For this review, take the finished solid that the model builds, in its own axes (mm). A direction names the side the tool comes from. Coordinates: 2 decimals unless noted, no trailing zeros. Loops run counter-clockwise (first coordinate to the right, second up) from the corner with the lowest first, then second, coordinate; pieces in that order, holes last. Notation, with made-up numbers: (1, 28) - (34, 28) arc R30 ccw to (34, 67) - close; hole circle Ø9 at (28, 69). An arc over 180 degrees is marked (long way). Answer as a JSON object with one key per item and string values. Group by question number.
Item 1: We need section B-B (y = -6). Give the boundary of the cut face in (x, z).
Item 2: We need section D-D (y = 9). Give the boundary of the cut face in (x, z).
Item 3: To check wall thickness, follow line 1 (X direction, y = 0, z = 5.2); line 2 (X direction, y = -10, z = 4.15); line 3 (Y direction, x = 0, z = 8.25). State the ranges of each line that lie inside material, in increasing order.
Item 4: Clearance check with flat-ended pins moving along their axes: pin 1 (5.5 mm diameter, centred on x = -27, y = 7.5, fed in from -Z); pin 2 (1 mm diameter, centred on y = -17.5, z = 6, fed in from -X); pin 3 (0.5 mm diameter, centred on x = 12.5, z = 4, fed in from -Y); pin 4 (10 mm diameter, centred on x = -11.5, y = -6.5, fed in from +Z). State where each tip first meets the part, or that it passes through.
Item 5: We need section A-A (y = -15.5). Give the boundary of the cut face in (x, z).
Item 6: We need section C-C (x = 10). Give the boundary of the cut face in (y, z).
Item 7: Mouldability with a two-part tool opening along Y and no side actions: class faces 1 (the cylindrical face through (23.124, 12.865, 5.735)), 2 (the flat face through (29.65, -3, 6)), 3 (the flat face through (0, -23.2, 6)) as released by +Y, released by -Y, zero draft, split by the parting line, or undercut.
Item 8: Tool access review of faces 4 (the flat face through (27, -12.3, 6)), 5 (the cylindrical face through (0.4, -26.8, 6.1)), 6 (the flat face through (-25, 4, 4.65)), 7 (the flat face through (0, -25, 8.4)), 8 (the flat face through (-1.7, -25, 6)): name each direction out of +Z, -Z, +X, -X, +Y, -Y from which nothing blocks a thin tool from reaching the whole face with its end or side.
from build123d import *

# Parameters (mm, degrees)
SKETCH_W             = 58.5
SKETCH_H             = 42.5
PAD_DEPTH            = 5
SKETCH002_W          = 43.18
SKETCH002_H          = 32.1
POCKET_DEPTH         = 5.001
SKETCH003_W          = 44.7
SKETCH003_H          = 21
POCKET001_DEPTH      = 5.001
POCKET004_DEPTH      = 4
SKETCH009_W          = 4.2
SKETCH009_H          = 3
PAD002_DEPTH         = 4
POCKET017_DEPTH      = 29.251
POCKET017_DEPTH_BACK = 29.251
SKETCH008_R          = 1
PAD016_DEPTH         = 3.5
POCKET018_DEPTH      = 5.001
FILLET_R             = 2
FILLET001_R          = 3
FILLET002_R          = 6
POCKET020_DEPTH      = 30.251
POCKET020_DEPTH_BACK = 28.251
CHAMFER_SIZE         = 1
BODY_PLACEMENT_ANGLE = 180


with BuildPart() as part:
    # Sketch → Pad (new body)
    with BuildSketch(Plane.XY):
        with Locations((0, 18.75)):
            Rectangle(SKETCH_W, SKETCH_H)
    extrude(amount=PAD_DEPTH)

    # Sketch002 → Pocket (cut, through all)
    with BuildSketch(Plane.XY):
        with Locations((0, 23.95)):
            Rectangle(SKETCH002_W, SKETCH002_H)
    extrude(amount=POCKET_DEPTH, mode=Mode.SUBTRACT)

    # Sketch003 → Pocket001 (cut, through all)
    with BuildSketch(Plane.XY):
        with Locations((0, 29.5)):
            Rectangle(SKETCH003_W, SKETCH003_H)
    extrude(amount=POCKET001_DEPTH, mode=Mode.SUBTRACT)

    # Sketch006 → Pocket004 (cut)
    with BuildSketch(Plane.XY):
        Polygon((-30, 14), (-23, 14), (-23, 5.1), (23, 5.1), (23, 14), (30, 14), (30, -2.5), (-30, -2.5), align=None)
    extrude(amount=POCKET004_DEPTH, mode=Mode.SUBTRACT)

    # Sketch009 → Pad002 (join)
    with BuildSketch(Plane(origin=(0, 0, 4), x_dir=(1, 0, 0), z_dir=(0, 0, -1))):
        with Locations((0, -1.6)):
            Rectangle(SKETCH009_W, SKETCH009_H)
    extrude(amount=PAD002_DEPTH)

    # Sketch005 → Pocket017 (cut, two sides)
    with BuildSketch(Plane.YZ) as pocket017_sk:
        Polygon((22.3, 7.55), (22.3, 3.75), (38.15, 3.75), (40, 3.250139), (40, 2.050139), (38.15, 1.55), (22.3, 1.55), (22.3, -2.25), (45.66, -2.25), (45.66, 7.55), align=None)
    extrude(amount=-POCKET017_DEPTH, mode=Mode.SUBTRACT)
    extrude(pocket017_sk.sketch, amount=POCKET017_DEPTH_BACK, mode=Mode.SUBTRACT)

    # Sketch008 (on Face13 of Pocket017) → Pad016 (join)
    with BuildSketch(Plane(origin=(0, 0, 4), x_dir=(1, 0, 0), z_dir=(0, 0, -1))):
        with Locations((0, -0.5)):
            Circle(SKETCH008_R)
    extrude(amount=PAD016_DEPTH)

    # Sketch034 → Pocket018 (cut, through all)
    with BuildSketch(Plane.XY):
        Polygon((-19, 0), (-1, 0), (-1, -3), (1, -3), (1, 0), (19, 0), (26.75, 2.820769), (26.75, 13.820769), (30, 13.820769), (30, -4), (-30, -4), (-30, 13.820769), (-26.75, 13.820769), (-26.75, 2.820769), align=None)
    extrude(amount=POCKET018_DEPTH, mode=Mode.SUBTRACT)

    # Fillet
    fillet_edges = [part.edges().sort_by_distance(p)[0] for p in [
        (29.25, 40, 2.650139),
        (22.35, 40, 2.650139),
        (-22.35, 40, 2.650139),
        (-29.25, 40, 2.650139),
    ]]
    fillet(fillet_edges, radius=FILLET_R)

    # Fillet001
    fillet001_edges = [part.edges().sort_by_distance(p)[0] for p in [
        (26.75, 2.820769, 4.5),
        (-26.75, 2.820769, 4.5),
    ]]
    fillet(fillet001_edges, radius=FILLET001_R)

    # Fillet002
    fillet002_edges = [part.edges().sort_by_distance(p)[0] for p in [
        (-19, 0, 4.5),
        (19, 0, 4.5),
    ]]
    fillet(fillet002_edges, radius=FILLET002_R)

    # Sketch038 (on Face7 of Fillet002) → Pocket020 (cut, two sides)
    with BuildSketch(Plane.YZ.offset(1)) as pocket020_sk:
        Polygon((-2.5, 4), (-1.461179, 5), (-1.461179, 5.705107), (-3.685712, 5.705107), (-3.685712, 4.047004), align=None)
    extrude(amount=-POCKET020_DEPTH, mode=Mode.SUBTRACT)
    extrude(pocket020_sk.sketch, amount=POCKET020_DEPTH_BACK, mode=Mode.SUBTRACT)

    # Chamfer
    chamfer_edges = [part.edges().sort_by_distance(p)[0] for p in [
        (-25.8, 22.3, 0),
        (-25.8, 22.3, 5),
        (25.8, 22.3, 5),
        (25.8, 22.3, 0),
    ]]
    chamfer(chamfer_edges, length=CHAMFER_SIZE)


with BuildPart() as part_1:
    # Body placement: moved
    add(part.part.moved(Location((0.4, -26.3, 8.4))).rotate(Axis((0.4, -26.3, 8.4), (0, 1, 0)), BODY_PLACEMENT_ANGLE))


solid = part_1.part
Check sheet entries:
{
 "1": {"outline": "(-28.85, 3.4) - (-21.95, 3.4) - (-21.95, 8.4) - (-28.85, 8.4) - close; (22.75, 3.4) - (29.65, 3.4) - (29.65, 8.4) - (22.75, 8.4) - close"},
 "2": {"outline": "(-28.85, 4.65) - (-21.95, 4.65) - (-21.95, 6.85) - (-28.85, 6.85) - close; (22.75, 4.65) - (29.65, 4.65) - (29.65, 6.85) - (22.75, 6.85) - close"},
 "3": {"line 1": "x = -28.85 to -21.95, 22.75 to 29.65", "line 2": "x = -28.85 to -21.19, 21.99 to 29.65", "line 3": "y = -26.2 to -23.2, -21.2 to -18.4"},
 "4": {"pin 1": "stops at z = 4.65", "pin 2": "stops at x = -22.6", "pin 3": "stops at y = -26.3", "pin 4": "passes through"},
 "5": {"outline": "(-26.35, 3.4) - (-21.19, 3.4) - (-21.19, 8.4) - (-22.6, 8.4) - (-22.6, 4.4) - (-26.35, 4.4) - close; (21.99, 3.4) - (27.15, 3.4) - (27.15, 4.4) - (23.4, 4.4) - (23.4, 8.4) - (21.99, 8.4) - close"},
 "6": {"outline": "(-26.3, 3.4) - (-18.4, 3.4) - (-18.4, 8.4) - (-21.2, 8.4) - (-21.2, 4.4) - (-26.3, 4.4) - close"},
 "7": {"face 1": "released by +Y", "face 2": "zero draft", "face 3": "undercut"},
 "8": {"face 4": "+Z, +X, -Y", "face 5": "+Z, -Y", "face 6": "-Z, +X, -X, +Y", "face 7": "+Z, +X, -X, +Y, -Y", "face 8": "+Z, -X, -Y"}
}
